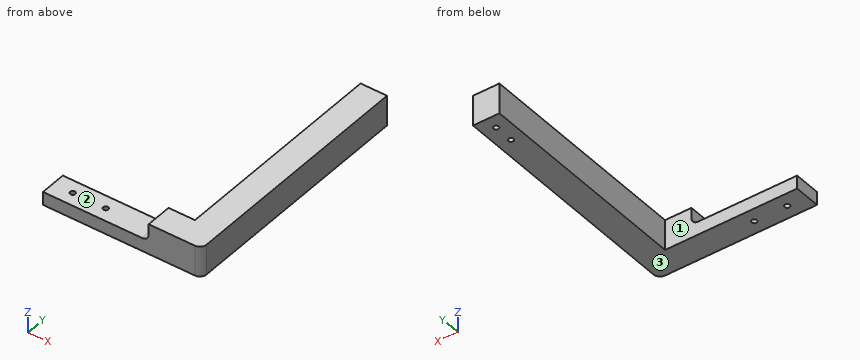
```python
from build123d import *

# Parameters (mm, degrees)
SKETCH_1_W          = 100
SKETCH_1_H          = 20
SKETCH_1_R          = 1.95
EXTRUDE_1_DEPTH     = 10
SKETCH_2_W          = 20
SKETCH_2_H          = 20
EXTRUDE_2_DEPTH     = 13
SKETCH_4_W          = 20
SKETCH_4_H          = 23
EXTRUDE_3_DEPTH     = 187
FILLET_2_R          = 5
FILLET_3_R          = 5
SKETCH_5_R          = 1.925
CUT_EXTRUDE_1_DEPTH = 5


with BuildPart() as part:
    # 草圖1 → 填料-伸長1 (new body)
    with BuildSketch(Plane.XY):
        with Locations((50, 10)):
            Rectangle(SKETCH_1_W, SKETCH_1_H)
        with Locations((15, 10)):
            Circle(SKETCH_1_R, mode=Mode.SUBTRACT)
        with Locations((40, 10)):
            Circle(SKETCH_1_R, mode=Mode.SUBTRACT)
    extrude(amount=EXTRUDE_1_DEPTH)

    # 草圖2 → 填料-伸長2 (add)
    with BuildSketch(Plane.XY.offset(10)):
        with Locations((90, 10)):
            Rectangle(SKETCH_2_W, SKETCH_2_H)
    extrude(amount=EXTRUDE_2_DEPTH)

    # 草圖4 → 填料-伸長3 (add)
    with BuildSketch(Plane.XZ):
        with Locations((110, 11.5)):
            Rectangle(SKETCH_4_W, SKETCH_4_H)
    extrude(amount=-EXTRUDE_3_DEPTH)

    # 圓角2
    fillet_2_edges = [part.edges().sort_by_distance(p)[0] for p in [
        (80, 10, 10),
    ]]
    fillet(fillet_2_edges, radius=FILLET_2_R)

    # 圓角3
    fillet_3_edges = [part.edges().sort_by_distance(p)[0] for p in [
        (120, 0, 11.5),
    ]]
    fillet(fillet_3_edges, radius=FILLET_3_R)

    # 草圖5 → 除料-伸長1 (cut)
    with BuildSketch(Plane.XY):
        with Locations((110, 177)):
            Circle(SKETCH_5_R)
        with Locations((110, 162)):
            Circle(SKETCH_5_R)
    extrude(amount=CUT_EXTRUDE_1_DEPTH, mode=Mode.SUBTRACT)


solid = part.part
```
Verification items for the finished model (mm, model axes). Face numbers are marked on the shaded views. A direction names the side the tool comes from. Round coordinates to 2 decimals unless told otherwise and drop trailing zeros. Write each loop counter-clockwise with the first axis right and the second up, starting at its lowest first coordinate (ties: lowest second). Pieces come first, ordered by that corner, then holes.
1. Section check D-D on y = 177. Enter the section's corners in (x, z) (3 decimals).
2. Section check A-A on x = 15. Enter the section's corners in (y, z).
3. Gauge pin test, flat ends, axial feed: P1, Ø1.9, axis at x = 109.5, y = 177.5, coming from the -Z side; P2, Ø7, axis at y = 106, z = 14, coming from the -X side; P3, Ø22, axis at x = 21, y = 14, coming from the +Z side. Record the tip position at first contact, or that the pin passes through.
4. Scan lines: L1, parallel to Y at x = 110, z = 2.4 (3 decimals); L2, parallel to X at y = 162, z = 3.45 (3 decimals); L3, parallel to Y at x = 40, z = 5.75. Record each from-to range of solid material in increasing order.
5. Access from +Z, -Z, +X, -X, +Y, -Y to the whole of each face (thin tool, end or side, straight path). Record for the marked faces 1, 2 and 3.
6. Section check B-B on y = 10. Enter the section's corners in (x, z), plus the area to 3 significant figures.
7. Section check C-C on z = 2. Enter the section's corners in (x, y) (3 decimals), plus the area to 3 significant figures.
Answer:
1. outline: (100, 0) - (108.075, 0) - (108.075, 5) - (111.925, 5) - (111.925, 0) - (120, 0) - (120, 23) - (100, 23) - close
2. outline: (0, 0) - (8.05, 0) - (8.05, 10) - (0, 10) - close; (11.95, 0) - (20, 0) - (20, 10) - (11.95, 10) - close
3. P1: stops at z = 5
3. P2: stops at x = 100
3. P3: stops at z = 10
4. L1: y = 0 to 160.075, 163.925 to 175.075, 178.925 to 187
4. L2: x = 100 to 108.075, 111.925 to 120
4. L3: y = 0 to 8.05, 11.95 to 20
5. face 1: +Z, -Z, -X, +Y
5. face 2: +Z, -X, +Y, -Y
5. face 3: -Z, +X, -X, +Y, -Y
6. outline: (0, 0) - (13.05, 0) - (13.05, 10) - (0, 10) - close; (16.95, 0) - (38.05, 0) - (38.05, 10) - (16.95, 10) - close; (41.95, 0) - (120, 0) - (120, 23) - (80, 23) - (80, 15) arc R5 cw to (75, 10) - (41.95, 10) - close
6. area: 1,650 mm2
7. outline: (0, 0) - (115, 0) arc R5 ccw to (120, 5) - (120, 187) - (100, 187) - (100, 20) - (0, 20) - close; hole circle Ø3.9 at (15, 10); hole circle Ø3.9 at (40, 10); hole circle Ø3.85 at (110, 162); hole circle Ø3.85 at (110, 177)
7. area: 5,690 mm2
